Source: CAD feature listing. Evaluate the final solid. Frame: model axes, mm. Give positions to 0.01 mm unless a question says otherwise; leave off trailing zeros. Loops run counter-clockwise (first coordinate to the right, second up) from the corner with the lowest first, then second, coordinate; pieces in that order, holes last.
from build123d import *

# Parameters (mm, degrees)
SKETCH1_R           = 50.8
BOSS_EXTRUDE1_DEPTH = 12.7
SKETCH2_R           = 3.175
SKETCH2_R_2         = 2.38125
SKETCH2_R_3         = 1.5875
CUT_EXTRUDE1_DEPTH  = 73.955945611
FILLET1_R           = 2.54


with BuildPart() as part:
    # Sketch1 → Boss-Extrude1 (new body)
    with BuildSketch(Plane(origin=(0, 0, 0), x_dir=(1, 0, 0), z_dir=(0, 1, 0))):
        with Locations(Location((0, 0, 0), (0, 0, 270))):
            Circle(SKETCH1_R)
    extrude(amount=BOSS_EXTRUDE1_DEPTH)

    # Sketch2 → Cut-Extrude1 (cut, through all)
    with BuildSketch(Plane(origin=(0, 12.7, 0), x_dir=(1, 0, 0), z_dir=(0, 1, 0))):
        with BuildLine():
            Line((5.844661521, -11.275190983), (3.175, -41.789561795))
            ThreePointArc((3.175, -41.789561795), (36.295124673, -20.955), (37.778322127, 18.14515024))
            Line((37.778322127, 18.14515024), (12.686932584, 0.575970138))
            ThreePointArc((12.686932584, 0.575970138), (10.998522628, -6.35), (5.844661521, -11.275190983))
        make_face()
        with BuildLine():
            ThreePointArc((-37.778322127, 18.14515024), (-36.295124673, -20.955), (-3.175, -41.789561795))
            Line((-3.175, -41.789561795), (-5.844661521, -11.275190983))
            ThreePointArc((-5.844661521, -11.275190983), (-10.998522628, -6.35), (-12.686932584, 0.575970138))
            Line((-12.686932584, 0.575970138), (-37.778322127, 18.14515024))
        make_face()
        with BuildLine():
            ThreePointArc((34.603322127, 23.644411554), (0, 41.91), (-34.603322127, 23.644411554))
            Line((-34.603322127, 23.644411554), (-6.842271064, 10.699220845))
            ThreePointArc((-6.842271064, 10.699220845), (-3.564400038, 12.189546848), (0, 12.7))
            ThreePointArc((0, 12.7), (3.564400038, 12.189546848), (6.842271064, 10.699220845))
            Line((6.842271064, 10.699220845), (34.603322127, 23.644411554))
        make_face()
        with Locations(Location((0, -19.05, 0), (0, 0, 270))):
            Circle(SKETCH2_R)
        with Locations(Location((0, -27.94, 0), (0, 0, 270))):
            Circle(SKETCH2_R_2)
        with Locations(Location((0, -36.83, 0), (0, 0, 270))):
            Circle(SKETCH2_R_3)
        with Locations(Location((-16.497783942, 9.525, 0), (0, 0, 270))):
            Circle(SKETCH2_R)
        with Locations(Location((-24.196749782, 13.97, 0), (0, 0, 270))):
            Circle(SKETCH2_R_2)
        with Locations(Location((-31.895715621, 18.415, 0), (0, 0, 270))):
            Circle(SKETCH2_R_3)
        with Locations(Location((16.497783942, 9.525, 0), (0, 0, 270))):
            Circle(SKETCH2_R)
        with Locations(Location((24.196749782, 13.97, 0), (0, 0, 270))):
            Circle(SKETCH2_R_2)
        with Locations(Location((31.895715621, 18.415, 0), (0, 0, 270))):
            Circle(SKETCH2_R_3)
    extrude(amount=-CUT_EXTRUDE1_DEPTH, mode=Mode.SUBTRACT)

    # Fillet1
    fillet1_edges = [part.edges().sort_by_distance(p)[0] for p in [
        (-12.686932584, 6.35, -0.575970138),
        (-5.844661521, 6.35, 11.275190983),
        (-3.175, 6.35, 41.789561795),
        (3.175, 6.35, 41.789561795),
        (5.844661521, 6.35, 11.275190983),
        (12.686932584, 6.35, -0.575970138),
        (37.778322127, 6.35, -18.14515024),
        (-34.603322127, 6.35, -23.644411554),
        (34.603322127, 6.35, -23.644411554),
        (6.842271064, 6.35, -10.699220845),
        (-6.842271064, 6.35, -10.699220845),
        (-37.778322127, 6.35, -18.14515024),
    ]]
    fillet(fillet1_edges, radius=FILLET1_R)


solid = part.part
1) Cut plane D-D (y = 11). State how many separate pieces and enclosed holes the cut face has, and give its area (3 significant figures).
Checks:
separate pieces: 1
enclosed holes: 12
area: 3,730 mm2
2) Pull-direction query (X, two-part tool) for faces 1 (the cylindrical face through (-19.6, 6.4, -10.2)), 2 (the cylindrical face through (-30.911, 6.261, -40.313)), 3 (the flat face through (1, 0, -1)); classes: released by +X, released by -X, zero draft, split by the parting line, or undercut.
Checks:
face 1: undercut
face 2: split by the parting line
face 3: zero draft
3) Cut plane C-C (z = -13.97). Return loops of the section in (x, y).
Checks:
outline: (-48.84, 0) - (-39.51, 0) - (-39.51, 12.7) - (-48.84, 12.7) - close; (-31.82, 0) - (-26.58, 0) - (-26.58, 12.7) - (-31.82, 12.7) - close; (-21.82, 0) - (-13.86, 0) - (-13.86, 12.7) - (-21.82, 12.7) - close; (13.86, 0) - (21.82, 0) - (21.82, 12.7) - (13.86, 12.7) - close; (26.58, 0) - (31.82, 0) - (31.82, 12.7) - (26.58, 12.7) - close; (39.51, 0) - (48.84, 0) - (48.84, 12.7) - (39.51, 12.7) - close
4) Contact query for flat-ended pins moving along their axis: P1, Ø4, axis at x = 36, y = 7.5, coming from the +Z side; P2, Ø4, axis at x = -11.5, y = 2, coming from the +Z side; P3, Ø1.5, axis at y = 10.5, z = 39.5, coming from the +X side. Output: stop coordinate, or through.
Checks:
P1: stops at z = 37.74
P2: stops at z = 49.9
P3: stops at x = 32.85
5) Ray query, probe 1 along X at (y, z) = (11.75, 18); probe 2 along X at (y, z) = (7.5, -13.5); probe 3 along Z at (x, y) = (2.5, 7). Return the intervals inside material, ascending.
Checks:
probe 1: x = -47.5 to -37.85, -5.26 to -3, 3 to 5.26, 37.85 to 47.5
probe 2: x = -48.97 to -39.68, -31.14 to -26.53, -21.86 to -12.85, 12.85 to 21.86, 26.53 to 31.14, 39.68 to 48.97
probe 3: z = -50.74 to -41.84, -12.45 to 17.09, 21.01 to 50.74
6) Cut plane B-B (x = -23). Return loops of the section in (y, z).
Checks:
outline: (0, -45.3) - (12.7, -45.3) - (12.7, -35.03) - (0, -35.03) - close; (0, -18.23) - (12.7, -18.23) - (12.7, -16.03) - (0, -16.03) - close; (0, -11.91) - (12.7, -11.91) - (12.7, -7.8) - (0, -7.8) - close; (0, 35.03) - (12.7, 35.03) - (12.7, 45.3) - (0, 45.3) - close
7) Cut plane A-A (z = 27.94). Return loops of the section in (x, y).
Checks:
outline: (-42.43, 0) - (-31.24, 0) - (-31.24, 12.7) - (-42.43, 12.7) - close; (-4.39, 0) - (-2.38, 0) - (-2.38, 12.7) - (-4.39, 12.7) - close; (2.38, 0) - (4.39, 0) - (4.39, 12.7) - (2.38, 12.7) - close; (31.24, 0) - (42.43, 0) - (42.43, 12.7) - (31.24, 12.7) - close
